```python
from build123d import *

# Parameters (mm, degrees)
F0_R     = 19.05
F1_DEPTH = 381
F2_R     = 17.78
F3_DEPTH = 381
F4_R     = 12.7
F5_DEPTH = 127
F6_R     = 11.43
F7_DEPTH = 127
F8_R     = 12.7
F9_DEPTH = 25.4


with BuildPart() as f1:
    # F0 (on Top) → F1 (new body)
    with BuildSketch(Plane.XY):
        Circle(F0_R)
    extrude(amount=F1_DEPTH)

    # F2 (on face) → F3 (cut)
    with BuildSketch(Plane.XY.offset(381)):
        Circle(F2_R)
    extrude(amount=-F3_DEPTH, mode=Mode.SUBTRACT)

    # F4 (on Right) → F5 (join)
    with BuildSketch(Plane.YZ):
        with Locations((-0.138039, 361.95)):
            Circle(F4_R)
    extrude(amount=F5_DEPTH)

    # F6 (on face) → F7 (cut)
    with BuildSketch(Plane.YZ.offset(127)):
        with Locations((0, 361.95)):
            Circle(F6_R)
    extrude(amount=-F7_DEPTH, mode=Mode.SUBTRACT)

    # F8 (on Right) → F9 (cut)
    with BuildSketch(Plane.YZ):
        with Locations((0.0001, 361.95)):
            Circle(F8_R)
    extrude(amount=-F9_DEPTH, mode=Mode.SUBTRACT)


solid = f1.part
```
Source: CAD feature listing. Evaluate the final solid. Frame: model axes, mm. A direction names the side the tool comes from. Round coordinates to 2 decimals unless told otherwise and drop trailing zeros. Loops run counter-clockwise (first coordinate to the right, second up) from the corner with the lowest first, then second, coordinate; pieces in that order, holes last. Notation, with made-up numbers: M -25.75,85.25 L 24.25,85.25 A5 cw 24.25,90.25 Z; hole C 50.5,62.25 d8. An arc over 180 degrees is marked long. Use a Markdown table: item, result. Add a question column.
1. Mould query, pull axis X, two halves, no side actions, for faces 6 (the flat face through (-16, 9, 381)), 7 (the cylindrical face through (-2.48, 18.888, 187.833)), 8 (the cylindrical face through (16.424, -6.81, 193.167)), 9 (the flat face through (127, -11, 357)). Classes: pulls with the +X half, pulls with the -X half, needs draft (parallel to the pull), parting line crosses it, or undercut.
2. Contact query for flat-ended pins moving along their axis: P1, Ø1.5, axis at x = 31.5, y = 11.5, coming from the -Z side; P2, Ø1, axis at y = 5, z = 186.5, coming from the +X side; P3, Ø10, axis at x = 28, y = 5, coming from the -Z side. Output: stop coordinate, or through.
3. Reachability of faces 1 (the flat face through (-16, 9, 0)), 2 (the cylindrical face through (64.389, -1.488, 373.283)), 3 (the cylindrical face through (6.8, 11.6, 357.1)), 4 (the cylindrical face through (-15.74, 8.85, 371.06)), 5 (the cylindrical face through (69.75, -2.89, 349.55)) from +Z, -Z, +X, -X, +Y, -Y: full face, straight path, thin tool, end or side. Return the list, or none.
4. Section query B-B on z = 361.95. Return the cut outline in (x, y), then the cut area to 3 significant figures.
5. Section query C-C on z = 150. Return the cut outline in (x, y).
6. Section query D-D on x = 77. Return the cut outline in (y, z), then the cut area to 3 significant figures.
7. Section query A-A on y = -7. Return the cut outline in (x, z).
8. Line query: line 1 (Y direction, x = 0, z = 224); line 2 (X direction, y = -1.5, z = 50.5); line 3 (Z direction, x = 62, y = 0). Output: solid intervals per line, ascending.
Reported:
| question | item | result |
|---|---|---|
| 1 | face 6 | needs draft |
| 1 | face 7 | parting line crosses it |
| 1 | face 8 | undercut |
| 1 | face 9 | pulls with the +X half |
| 2 | P1 | stops at z = 355.41 |
| 2 | P2 | stops at x = 18.51 |
| 2 | P3 | stops at z = 349.25 |
| 3 | face 1 | -Z, +X, -X, +Y, -Y |
| 3 | face 2 | +X, -X |
| 3 | face 3 | none |
| 3 | face 4 | -X |
| 3 | face 5 | +X |
| 4 | outline | M -14.2,-12.7 A19.05 ccw 14.07,-12.84 L 127,-12.84 L 127,-11.43 L 0,-11.43 L 0,-12.84 L 12.3,-12.84 A17.78 cw -12.44,-12.7 Z; M -14.2,12.7 L -12.44,12.7 A17.78 cw 12.58,12.56 L 0,12.56 L 0,11.43 L 127,11.43 L 127,12.56 L 14.32,12.56 A19.05 ccw Z |
| 4 | area | 398 mm² |
| 5 | outline | C 0,0 d38.1; hole C 0,0 d35.56 |
| 6 | outline | C -0.14,361.95 d25.4; hole C 0,361.95 d22.86 |
| 6 | area | 96.3 mm² |
| 7 | outline | M -17.72,0 L -16.34,0 L -16.34,351.35 L -17.72,351.35 Z; M -17.72,372.55 L -16.34,372.55 L -16.34,381 L -17.72,381 Z; M 0,351.26 L 16.34,351.26 L 16.34,0 L 17.72,0 L 17.72,351.26 L 127,351.26 L 127,352.91 L 0,352.91 Z; M 0,370.99 L 127,370.99 L 127,372.64 L 17.72,372.64 L 17.72,381 L 16.34,381 L 16.34,372.64 L 0,372.64 Z |
| 8 | line 1 | y = -19.05 to -17.78, 17.78 to 19.05 |
| 8 | line 2 | x = -18.99 to -17.72, 17.72 to 18.99 |
| 8 | line 3 | z = 349.25 to 350.52, 373.38 to 374.65 |
